The listing builds one solid part. Answer for the finished solid, in the listing's coordinates (mm). Face numbers are marked on the shaded views. A direction names the side the tool comes from. Round coordinates to 2 decimals unless told otherwise and drop trailing zeros. Loops run counter-clockwise (first coordinate to the right, second up) from the corner with the lowest first, then second, coordinate; pieces in that order, holes last. Notation, with made-up numbers: (41.5, 2.25) -> (98.5, 2.25) arc R18 ccw to (98.5, 22.25) -> close; hole circle Ø9 at (17.5, 84). An arc over 180 degrees is marked (long way). Use a Markdown table: item, result. Add a question column.
Q1. Section A-A on y = 24 is taken. Give the vertices of the cut face in (x, z).
Q2. Which of the six approach directions +Z, -Z, +X, -X, +Y, -Y give full straight-line access (tool end or side, diameter ignored) to the marked faces 1 and 2?
Q3. Section C-C on x = -22 is taken. Give the vertices of the cut face in (y, z), then the cut area to 3 significant figures.
Q4. Consider line 1 (Y direction, x = -20, z = 21.75); line 2 (Y direction, x = 9, z = 13.75); line 3 (X direction, y = 24, z = 26.75). Determine where each line is inside the solid, lowest interval first.
Q5. Section B-B on z = 13.5 is taken. Give the vertices of the cut face in (x, y).
Q6. Given pin 1 Ø5 at (x, y) = (-12, -23.5) entering from +Z; pin 2 Ø20 at (x, y) = (10, 18) entering from +Z, each flat-ended and moving along its own axis, determine where each tip first touches the part or whether it passes through.
Q7. Section D-D on z = 26.5 is taken. Give the vertices of the cut face in (x, y), then the cut area to 3 significant figures.
from build123d import *

# Parameters (mm, degrees)
PAD_DEPTH       = 30
POCKET_DEPTH    = 12
POCKET001_DEPTH = 20


with BuildPart() as part:
    # Sketch001 → Pad (new body)
    with BuildSketch(Plane.XY):
        with BuildLine():
            Line((-60, 30), (-60, -30))
            ThreePointArc((-60, -30), (-57.071068, -37.071068), (-50, -40))
            Line((-50, -40), (50, -40))
            ThreePointArc((50, -40), (57.071068, -37.071068), (60, -30))
            Line((60, -30), (60, 30))
            ThreePointArc((60, 30), (57.071068, 37.071068), (50, 40))
            Line((50, 40), (-50, 40))
            ThreePointArc((-50, 40), (-57.071068, 37.071068), (-60, 30))
        make_face()
    extrude(amount=PAD_DEPTH)

    # Binder → Pocket (cut)
    with BuildSketch(Plane(origin=(0, 20, 30), x_dir=(0, 1, 0), z_dir=(0, 0, 1))):
        with BuildLine():
            Line((7.5, 40), (-7.5, 40))
            ThreePointArc((-7.5, 40), (-11.035534, 38.535534), (-12.5, 35))
            Line((-12.5, 35), (-12.5, -35))
            ThreePointArc((-12.5, -35), (-11.035534, -38.535534), (-7.5, -40))
            Line((-7.5, -40), (7.5, -40))
            ThreePointArc((7.5, -40), (11.035534, -38.535534), (12.5, -35))
            Line((12.5, -35), (12.5, 35))
            ThreePointArc((12.5, 35), (11.035534, 38.535534), (7.5, 40))
        make_face()
    extrude(amount=-POCKET_DEPTH, mode=Mode.SUBTRACT)

    # Binder001 → Pocket001 (cut)
    with BuildSketch(Plane(origin=(0, -20, 30), x_dir=(0, 1, 0), z_dir=(0, 0, 1))):
        with BuildLine():
            Line((7.5, 40), (-7.5, 40))
            ThreePointArc((-7.5, 40), (-11.035534, 38.535534), (-12.5, 35))
            Line((-12.5, 35), (-12.5, -35))
            ThreePointArc((-12.5, -35), (-11.035534, -38.535534), (-7.5, -40))
            Line((-7.5, -40), (7.5, -40))
            ThreePointArc((7.5, -40), (11.035534, -38.535534), (12.5, -35))
            Line((12.5, -35), (12.5, 35))
            ThreePointArc((12.5, 35), (11.035534, 38.535534), (7.5, 40))
        make_face()
    extrude(amount=-POCKET001_DEPTH, mode=Mode.SUBTRACT)


solid = part.part
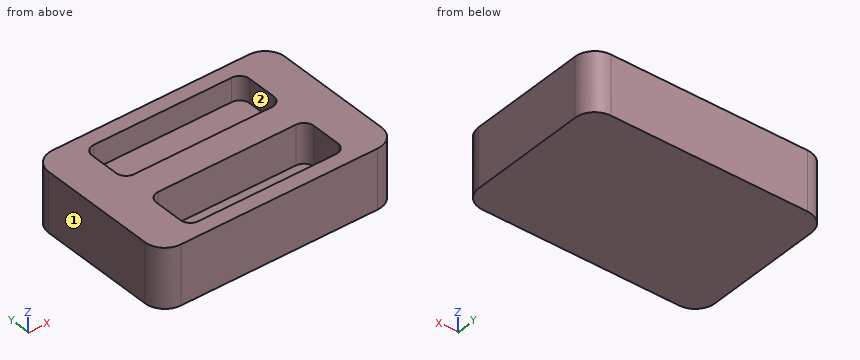
Checked values:
| question | item | result |
|---|---|---|
| 1 | outline | (-60, 0) -> (60, 0) -> (60, 30) -> (40, 30) -> (40, 18) -> (-40, 18) -> (-40, 30) -> (-60, 30) -> close |
| 2 | face 1 | +Z, -Z, -X, +Y, -Y |
| 2 | face 2 | +Z |
| 3 | outline | (-40, 0) -> (40, 0) -> (40, 30) -> (32.5, 30) -> (32.5, 18) -> (7.5, 18) -> (7.5, 30) -> (-7.5, 30) -> (-7.5, 10) -> (-32.5, 10) -> (-32.5, 30) -> (-40, 30) -> close |
| 3 | area | 1,600 mm2 |
| 4 | line 1 | y = -40 to -32.5, -7.5 to 7.5, 32.5 to 40 |
| 4 | line 2 | y = -40 to -32.5, -7.5 to 40 |
| 4 | line 3 | x = -60 to -40, 40 to 60 |
| 5 | outline | (-60, -30) arc R10 ccw to (-50, -40) -> (50, -40) arc R10 ccw to (60, -30) -> (60, 30) arc R10 ccw to (50, 40) -> (-50, 40) arc R10 ccw to (-60, 30) -> close; hole (-40, -27.5) arc R5 ccw to (-35, -32.5) -> (35, -32.5) arc R5 ccw to (40, -27.5) -> (40, -12.5) arc R5 ccw to (35, -7.5) -> (-35, -7.5) arc R5 ccw to (-40, -12.5) -> close |
| 6 | pin 1 | stops at z = 10 |
| 6 | pin 2 | stops at z = 18 |
| 7 | outline | (-60, -30) arc R10 ccw to (-50, -40) -> (50, -40) arc R10 ccw to (60, -30) -> (60, 30) arc R10 ccw to (50, 40) -> (-50, 40) arc R10 ccw to (-60, 30) -> close; hole (-40, -27.5) arc R5 ccw to (-35, -32.5) -> (35, -32.5) arc R5 ccw to (40, -27.5) -> (40, -12.5) arc R5 ccw to (35, -7.5) -> (-35, -7.5) arc R5 ccw to (-40, -12.5) -> close; hole (-40, 12.5) arc R5 ccw to (-35, 7.5) -> (35, 7.5) arc R5 ccw to (40, 12.5) -> (40, 27.5) arc R5 ccw to (35, 32.5) -> (-35, 32.5) arc R5 ccw to (-40, 27.5) -> close |
| 7 | area | 5,560 mm2 |
